Check sheet for the modelled part. Datum: model origin and axes. Units: mm. Round coordinates to 2 decimals unless told otherwise and drop trailing zeros. Write each loop counter-clockwise with the first axis right and the second up, starting at its lowest first coordinate (ties: lowest second). Pieces come first, ordered by that corner, then holes. Notation, with made-up numbers: (-5.5, 79) -> (34.5, 79) arc R25 cw to (34.5, 104) -> close; hole circle Ø2 at (50, 30.5). An arc over 180 degrees is marked (long way). Answer as a JSON object with one key per item and string values. Group by question number.
```python
from build123d import *

# Parameters (mm, degrees)
IZIM1_W                     = 78
IZIM1_H                     = 65
Y_KSEKLIK_EKSTR_ZYON1_DEPTH = 3
IZIM2_W                     = 3
IZIM2_H                     = 3
Y_KSEKLIK_EKSTR_ZYON2_DEPTH = 5
IZIM4_R                     = 1.25
Y_KSEKLIK_EKSTR_ZYON3_DEPTH = 5
IZIM5_R                     = 1.25
Y_KSEKLIK_EKSTR_ZYON4_DEPTH = 5
IZIM6_R                     = 2
KES_EKSTR_ZYON2_DEPTH       = 10


with BuildPart() as part:
    # Çizim1 → Yükseklik-Ekstrüzyon1 (new body)
    with BuildSketch(Plane.XY):
        with Locations((39, 32.5)):
            Rectangle(IZIM1_W, IZIM1_H)
    extrude(amount=Y_KSEKLIK_EKSTR_ZYON1_DEPTH)

    # Çizim2 → Yükseklik-Ekstrüzyon2 (add)
    with BuildSketch(Plane.ZY):
        with Locations((1.5, 56.5)):
            Rectangle(IZIM2_W, IZIM2_H)
        with Locations((1.5, 26.5)):
            Rectangle(IZIM2_W, IZIM2_H)
    extrude(amount=Y_KSEKLIK_EKSTR_ZYON2_DEPTH)

    # Çizim4 → Yükseklik-Ekstrüzyon3 (add)
    with BuildSketch(Plane.XZ.offset(-55)):
        with Locations(Location((-3, 1.5, 0), (0, 0, 90))):
            Circle(IZIM4_R)
    extrude(amount=Y_KSEKLIK_EKSTR_ZYON3_DEPTH)

    # Çizim5 → Yükseklik-Ekstrüzyon4 (add)
    with BuildSketch(Plane.XZ.offset(-25)):
        with Locations(Location((-3, 1.5, 0), (0, 0, 90))):
            Circle(IZIM5_R)
    extrude(amount=Y_KSEKLIK_EKSTR_ZYON4_DEPTH)

    # Çizim6 → Kes-Ekstrüzyon2 (cut)
    with BuildSketch(Plane.XY.offset(3)):
        with Locations((73, 5)):
            Circle(IZIM6_R)
    extrude(amount=-KES_EKSTR_ZYON2_DEPTH, mode=Mode.SUBTRACT)


solid = part.part
```
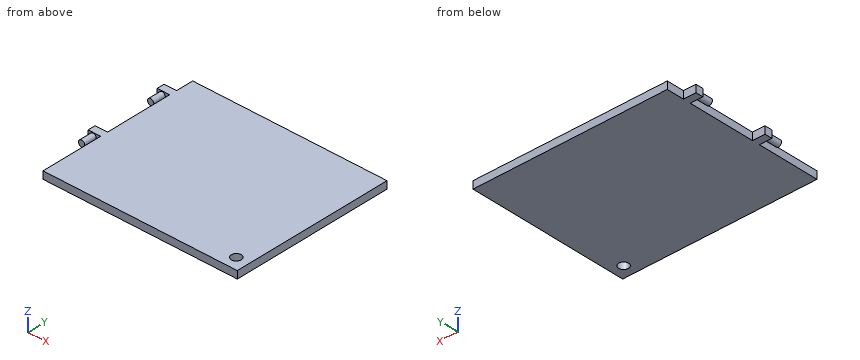
(1) Go/stop test with flat-tipped pins: pin 1 Ø0.8 at (x, z) = (-3.5, 1) entering from -Y; pin 2 Ø0.9 at (x, z) = (-2, 1.5) entering from +Y. Record where each tip stops, or that it passes through.
(2) Section check C-C on z = 1.5. Record the cut outline in (x, y).
(3) Section check B-B on y = 5. Record the cut outline in (x, z).
(4) Section check A-A on x = -3. Record the cut outline in (y, z), then the cut area to 3 significant figures.
(5) Scan lines: line 1 along Y through (x, z) = (73, 1.5); line 2 along X through (y, z) = (24, 2.6); line 3 along X through (y, z) = (33, 2.4). Record each from-to range of solid material in increasing order.
(6) Section check D-D on y = 19. Record the cut outline in (x, z).
Data:
{
 "1": {"pin 1": "stops at y = 20", "pin 2": "stops at y = 58"},
 "2": {"outline": "(-5, 25) -> (-4.25, 25) -> (-4.25, 20) -> (-1.75, 20) -> (-1.75, 25) -> (0, 25) -> (0, 0) -> (78, 0) -> (78, 65) -> (0, 65) -> (0, 58) -> (-5, 58) -> (-5, 55) -> (-4.25, 55) -> (-4.25, 50) -> (-1.75, 50) -> (-1.75, 55) -> (0, 55) -> (0, 28) -> (-5, 28) -> close; hole circle Ø4 at (73, 5)"},
 "3": {"outline": "(0, 0) -> (71, 0) -> (71, 3) -> (0, 3) -> close; (75, 0) -> (78, 0) -> (78, 3) -> (75, 3) -> close"},
 "4": {"outline": "(20, 0.25) -> (25, 0.25) -> (25, 0) -> (28, 0) -> (28, 3) -> (25, 3) -> (25, 2.75) -> (20, 2.75) -> close; (50, 0.25) -> (55, 0.25) -> (55, 0) -> (58, 0) -> (58, 3) -> (55, 3) -> (55, 2.75) -> (50, 2.75) -> close", "area": "43.0 mm²"},
 "5": {"line 1": "y = 0 to 3, 7 to 65", "line 2": "x = -3.59 to -2.41, 0 to 78", "line 3": "x = 0 to 78"},
 "6": {"outline": "(0, 0) -> (78, 0) -> (78, 3) -> (0, 3) -> close"}
}
